Verification items for the finished model (mm, model axes). Face numbers are marked on the shaded views. A direction names the side the tool comes from. Round coordinates to 2 decimals unless told otherwise and drop trailing zeros. Put each result on its own line as item: value.
from build123d import *

# Parameters (mm, degrees)
SKETCH1_R           = 1
BOSS_EXTRUDE1_DEPTH = 1
BOSS_EXTRUDE6_DEPTH = 2.5
FILLET6_R           = 1.5
FILLET7_R           = 2
CHAMFER1_SIZE       = 1


# Some blends are built 0.0001 mm under size
with BuildPart() as part:
    # Sketch1 → Boss-Extrude1 (new body)
    with BuildSketch(Plane.XY):
        Polygon((-13.5, 5.5), (-13.5, -5.5), (4.5, -5.5), (4.5, -3.5), (13.5, -3.5), (13.5, 5.5), align=None)
        with Locations((-11.5, -3.5)):
            Circle(SKETCH1_R, mode=Mode.SUBTRACT)
        with Locations((11.5, 3.5)):
            Circle(SKETCH1_R, mode=Mode.SUBTRACT)
    extrude(amount=BOSS_EXTRUDE1_DEPTH)

    # Sketch3 → Boss-Extrude6 (add, symmetric)
    with BuildSketch(Plane(origin=(0, 0, 0), x_dir=(0, 0, -1), z_dir=(1, 0, 0))):
        Polygon((-1, -3.5), (-6.5, -3.5), (-6.5, 4), (-1.5, 4), (-1.5, 2.5), (-5, 2.5), (-5, -2), (-1, -2), align=None)
    extrude(amount=BOSS_EXTRUDE6_DEPTH, both=True)

    # Fillet6
    fillet6_edges = [part.edges().sort_by_distance(p)[0] for p in [
        (0, -2, 1),
        (0, 2.5, 5),
        (0, -2, 5),
    ]]
    fillet(fillet6_edges, radius=FILLET6_R)

    # Fillet7
    fillet7_edges = [part.edges().sort_by_distance(p)[0] for p in [
        (0, -3.5, 6.5),
        (0, 4, 6.5),
    ]]
    fillet(fillet7_edges, radius=FILLET7_R)

    # Chamfer1
    chamfer1_edges = [part.edges().sort_by_distance(p)[0] for p in [
        (0, 5.5, 1),
    ]]
    chamfer(chamfer1_edges, length=CHAMFER1_SIZE - 0.0001)  # a hair under: the kernel refuses the full size
    chamfer1_2_edges = [part.edges().sort_by_distance(p)[0] for p in [
        (-4.5, -5.5, 1),
    ]]
    chamfer(chamfer1_2_edges, length=CHAMFER1_SIZE - 0.0001)  # a hair under: the kernel refuses the full size
    chamfer1_3_edges = [part.edges().sort_by_distance(p)[0] for p in [
        (-13.5, 0, 1),
    ]]
    chamfer(chamfer1_3_edges, length=CHAMFER1_SIZE - 0.0001)  # a hair under: the kernel refuses the full size
    chamfer1_4_edges = [part.edges().sort_by_distance(p)[0] for p in [
        (9, -3.5, 1),
    ]]
    chamfer(chamfer1_4_edges, length=CHAMFER1_SIZE - 0.0001)  # a hair under: the kernel refuses the full size
    chamfer1_5_edges = [part.edges().sort_by_distance(p)[0] for p in [
        (13.5, 1, 1),
    ]]
    chamfer(chamfer1_5_edges, length=CHAMFER1_SIZE - 0.0001)  # a hair under: the kernel refuses the full size
    chamfer1_6_edges = [part.edges().sort_by_distance(p)[0] for p in [
        (0, -3.5, 1),
    ]]
    chamfer(chamfer1_6_edges, length=CHAMFER1_SIZE)
    chamfer1_7_edges = [part.edges().sort_by_distance(p)[0] for p in [
        (-2.5, -2, 1),
    ]]
    chamfer(chamfer1_7_edges, length=CHAMFER1_SIZE)
    chamfer1_8_edges = [part.edges().sort_by_distance(p)[0] for p in [
        (2.5, -2, 1),
    ]]
    chamfer(chamfer1_8_edges, length=CHAMFER1_SIZE)
    chamfer1_9_edges = [part.edges().sort_by_distance(p)[0] for p in [
        (4.5, -4.00005, 1),
    ]]
    chamfer(chamfer1_9_edges, length=CHAMFER1_SIZE - 0.0001)  # a hair under: the kernel refuses the full size
    # the kernel refuses this chamfer: 1 mm, written as the material it takes off along each edge
    with BuildSketch(Plane(origin=(11.5, 3.5, 1), x_dir=(1, 0, 0), z_dir=(0, -1, 0))) as chamfer1_10_piece_1:
        with BuildLine():
            Line((2.028284271, 0.028284271), (0.971715729, -1.028284271))
            Line((0.971715729, -1.028284271), (0.951715729, -1.028284271))
            ThreePointArc((0.951715729, -1.028284271), (0.98, -0.514142136), (0.98, 0))
            Line((0.98, 0), (1, 0.02))
            ThreePointArc((1, 0.02), (1.514142136, 0.02), (2.028284271, 0.048284271))
            Line((2.028284271, 0.048284271), (2.028284271, 0.028284271))
        make_face()
    revolve(axis=Axis((11.5, 3.5, 1), (0, 0, 1)), mode=Mode.SUBTRACT)
    # the kernel refuses this chamfer: 1 mm, written as the material it takes off along each edge
    with BuildSketch(Plane(origin=(-11.5, -3.5, 1), x_dir=(1, 0, 0), z_dir=(0, -1, 0))) as chamfer1_11_piece_1:
        with BuildLine():
            Line((2.028284271, 0.028284271), (0.971715729, -1.028284271))
            Line((0.971715729, -1.028284271), (0.951715729, -1.028284271))
            ThreePointArc((0.951715729, -1.028284271), (0.98, -0.514142136), (0.98, 0))
            Line((0.98, 0), (1, 0.02))
            ThreePointArc((1, 0.02), (1.514142136, 0.02), (2.028284271, 0.048284271))
            Line((2.028284271, 0.048284271), (2.028284271, 0.028284271))
        make_face()
    revolve(axis=Axis((-11.5, -3.5, 1), (0, 0, 1)), mode=Mode.SUBTRACT)


solid = part.part
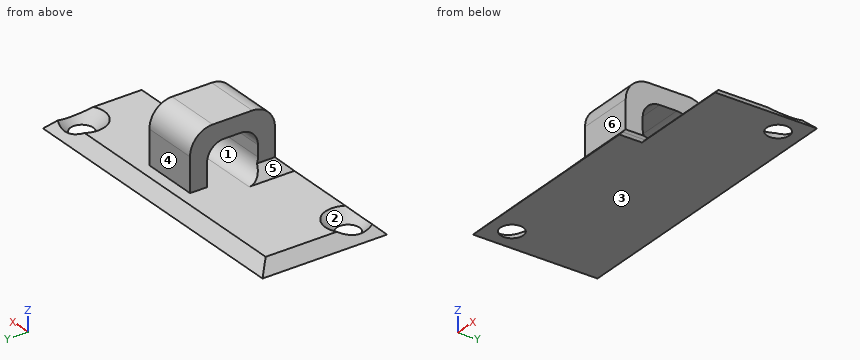
Item 1: Release check for a two-part mould opening along Z. For the marked faces 1, 2 and 3 record: +Z half, -Z half, draft (parallel to the pull), parting line (faces both ways), or undercut.
Check sheet entries:
face 1: undercut
face 2: +Z half
face 3: -Z half
Item 2: Gauge pin test, flat ends, axial feed: pin 1 Ø3 at (y, z) = (-1, 3.5) entering from +X; pin 2 Ø2.5 at (x, z) = (0, 3) entering from +Y; pin 3 Ø2 at (x, z) = (3.5, 2) entering from -Y; pin 4 Ø2.5 at (y, z) = (-0.5, 3) entering from -X. Record the tip position at first contact, or that the pin passes through.
Check sheet entries:
pin 1: stops at x = 2.5
pin 2: stops at y = 4
pin 3: stops at y = -4.5
pin 4: passes through
Item 3: Tool access check on the marked faces 4, 5 and 6. Record the directions out of +Z, -Z, +X, -X, +Y, -Y that give a thin tool (end or side, any length) a straight path to the whole face; none if there is none.
Check sheet entries:
face 4: +Z, +X, -X, +Y
face 5: +Z, -X, +Y, -Y
face 6: +Z, +X, -X, -Y
Item 4: Material ranges on L1, parallel to Z at x = -5, y = 4.25; L2, parallel to Y at x = 3.75, z = 0.5; L3, parallel to X at y = 3.25, z = 4.5, recorded low to high. Write a range as [from, to].
Check sheet entries:
L1: z = [0, 1]
L2: y = [-5, 5]
L3: x = [-2.5, 2.5]
Item 5: Section check B-B on y = 3.5. State how many separate pieces and enclosed holes the cut face has, then the cut area to 3 significant figures.
Check sheet entries:
separate pieces: 3
enclosed holes: 0
area: 44.9 mm^2
